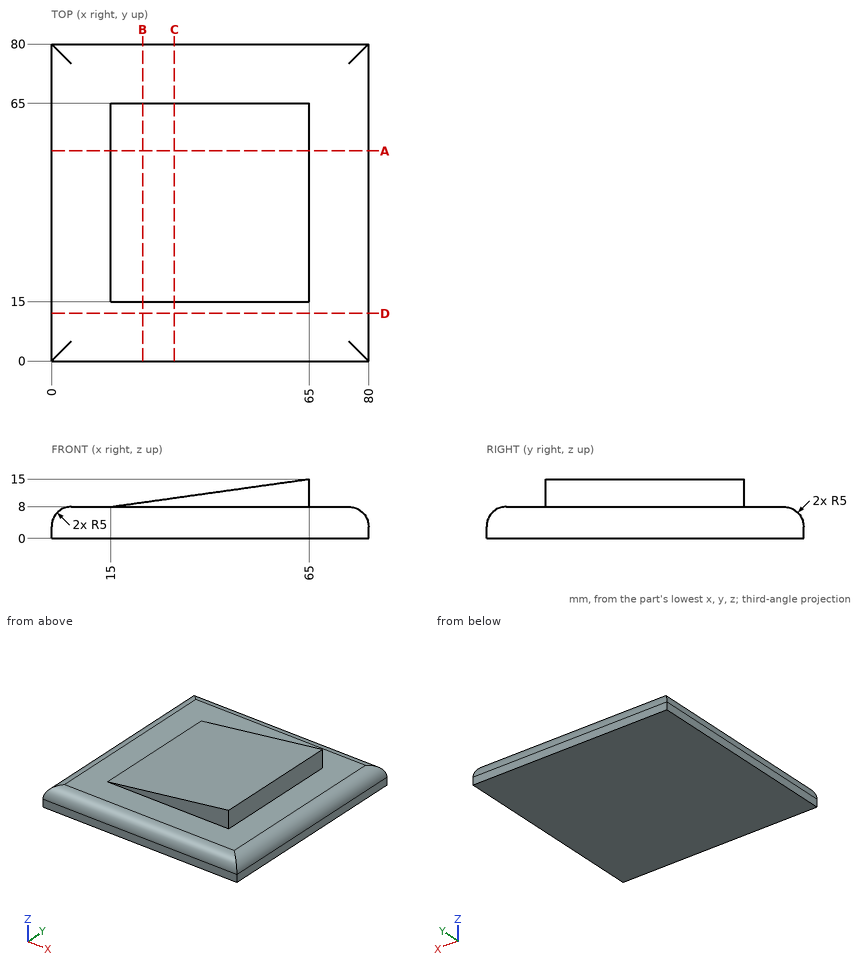
Design review of the part shown in the three views and the two pictorial views. Dimensions are in mm from the part's minimum x, y and z. Round coordinates to 2 decimals unless told otherwise and drop trailing zeros. Write each loop counter-clockwise with the first axis right and the second up, starting at its lowest first coordinate (ties: lowest second). Pieces come first, ordered by that corner, then holes.
Item 1: Wall thickness on L1, parallel to Z at x = 66.5, y = 18; L2, parallel to X at y = 45.5, z = 3.25; L3, parallel to Y at x = 20.5, z = 5: over which ranges is each line inside the solid? List them lowest first.
Item 2: Consider section D-D on y = 12. Give the boundary of the cut face in (x, z).
Item 3: Consider section A-A on y = 53. Give the boundary of the cut face in (x, z), and give its area (3 significant figures).
Item 4: Consider section B-B on x = 23. Give the boundary of the cut face in (y, z).
Item 5: Consider section C-C on x = 31. Give the boundary of the cut face in (y, z), and give its area (3 significant figures).
Item 6: For pin 1 Ø2 at (x, y) = (61.5, 24.5) entering from +Z; pin 2 Ø4 at (y, z) = (42.5, 7) entering from -X; pin 3 Ø3 at (x, z) = (49, 6.5) entering from +Y; pin 4 Ø12 at (x, y) = (68, 12) entering from -Z, all flat-tipped, find the tip position at first contact; note any pin that passes through.
Check values:
1. L1: z = 0 to 8
1. L2: x = 0.01 to 79.99
1. L3: y = 0.42 to 79.58
2. outline: (0, 0) - (80, 0) - (80, 3) arc R5 ccw to (75, 8) - (5, 8) arc R5 ccw to (0, 3) - close
3. outline: (0, 0) - (80, 0) - (80, 3) arc R5 ccw to (75, 8) - (65, 8) - (65, 15) - (15, 8) - (5, 8) arc R5 ccw to (0, 3) - close
3. area: 804 mm2
4. outline: (0, 0) - (80, 0) - (80, 3) arc R5 ccw to (75, 8) - (65, 8) - (65, 9.12) - (15, 9.12) - (15, 8) - (5, 8) arc R5 ccw to (0, 3) - close
5. outline: (0, 0) - (80, 0) - (80, 3) arc R5 ccw to (75, 8) - (65, 8) - (65, 10.24) - (15, 10.24) - (15, 8) - (5, 8) arc R5 ccw to (0, 3) - close
5. area: 741 mm2
6. pin 1: stops at z = 14.65
6. pin 2: stops at x = 0.42
6. pin 3: stops at y = 79.58
6. pin 4: stops at z = 0
